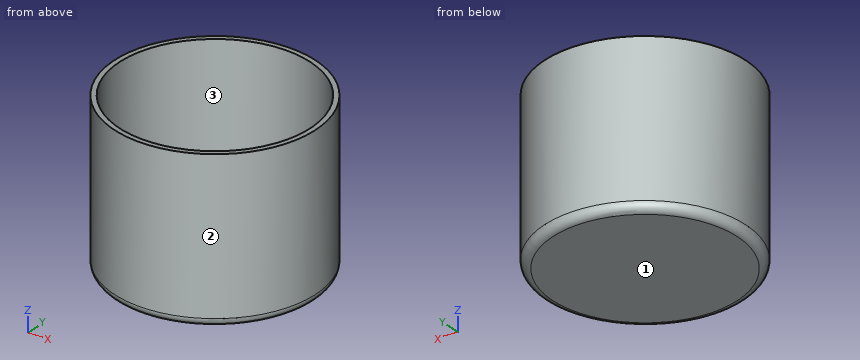
```python
from build123d import *

# Parameters (mm, degrees)
F3_DEPTH = 10


with BuildPart() as f1:
    # F0 (on Right) → F1 (revolve)
    with BuildSketch(Plane.YZ):
        with BuildLine():
            Line((0, 1.6), (0, 0))
            Line((0, 0), (29, 0))
            ThreePointArc((29, 0), (30.838478, 0.761522), (31.6, 2.6))
            Line((31.6, 2.6), (31.6, 50))
            Line((31.6, 50), (30, 50))
            Line((30, 50), (30, 2.6))
            ThreePointArc((30, 2.6), (29.707107, 1.892893), (29, 1.6))
            Line((29, 1.6), (4.2, 1.6))
            Line((4.2, 1.6), (4.2, 11.6))
            Line((4.2, 11.6), (2.6, 11.6))
            Line((2.6, 11.6), (2.6, 1.6))
            Line((2.6, 1.6), (0, 1.6))
        make_face()
    revolve(axis=Axis((0, 0, 0.8), (0, 0, 1)))

    # F2 (on face) → F3 (join, through all)
    with BuildSketch(Plane.XY.offset(11.6)):
        with BuildLine():
            ThreePointArc((1.385641, 2.2), (0, 2.6), (-1.385641, 2.2))
            Line((-1.385641, 2.2), (1.385641, 2.2))
        make_face()
    extrude(amount=-F3_DEPTH)


solid = f1.part
```
CAD build for the part. Positions are in the model's coordinates, mm. Face numbers are marked on the shaded views. Round coordinates to 2 decimals unless told otherwise and drop trailing zeros. Order: outer loops, then holes, each group sorted by start corner. A loop starts at its lowest first (then second) coordinate and runs counter-clockwise, first axis right, second up. Notation, with made-up numbers: (46, 16) - (72, 16) arc R28 ccw to (72, 50) - close; hole circle Ø3 at (88, 80). An arc over 180 degrees is marked (long way). Answer as CSV lines item,"result". Start each with the question number.
1. Saw through at C-C, the plane z = 23.5. Write the cut outline in (x, y).
2. Saw through at A-A, the plane z = 5.5. Write the cut outline in (x, y), and give its area (3 significant figures).
3. Saw through at B-B, the plane x = 0. Write the cut outline in (y, z), and give its area (3 significant figures).
4. Pin check, flat tips, straight feed: pin 1 (6 mm diameter, centred on y = -18.5, z = 40, fed in from -X); pin 2 (6.5 mm diameter, centred on x = 0, y = 0.5, fed in from +Z); pin 3 (2 mm diameter, centred on y = 4.5, z = 21.5, fed in from -X). Stop position of each tip, or through.
5. Saw through at D-D, the plane y = 0. Write the cut outline in (x, z), and give its area (3 significant figures).
6. Drill centre lines: L1, parallel to X at y = 0, z = 6; L2, parallel to Y at x = 0, z = 5; L3, parallel to X at y = 3, z = 10. Where is each one in solid material? Low to high. Write a range as [from, to].
7. Pull direction X, two halves, no side cores. Call the marked faces 1, 2 and 3: +X half, -X half, draft (parallel to the pull), parting line (faces both ways), or undercut.
Model answer:
1,outline,"circle Ø63.2 at (0, 0); hole circle Ø60 at (0, 0)"
2,outline,"circle Ø63.2 at (0, 0); circle Ø8.4 at (0, 0); hole circle Ø60 at (0, 0); hole (-1.39, 2.2) arc R2.6 ccw (long way) to (1.39, 2.2) - close"
2,area,"345 mm²"
3,outline,"(-31.6, 2.6) arc R2.6 ccw to (-29, 0) - (29, 0) arc R2.6 ccw to (31.6, 2.6) - (31.6, 50) - (30, 50) - (30, 2.6) arc R1 cw to (29, 1.6) - (4.2, 1.6) - (4.2, 11.6) - (2.2, 11.6) - (2.2, 1.6) - (-2.6, 1.6) - (-2.6, 11.6) - (-4.2, 11.6) - (-4.2, 1.6) - (-29, 1.6) arc R1 cw to (-30, 2.6) - (-30, 50) - (-31.6, 50) - close"
3,area,"290 mm²"
4,pin 1,"stops at x = -27.54"
4,pin 2,"stops at z = 11.6"
4,pin 3,"stops at x = -31.41"
5,outline,"(-31.6, 2.6) arc R2.6 ccw to (-29, 0) - (29, 0) arc R2.6 ccw to (31.6, 2.6) - (31.6, 50) - (30, 50) - (30, 2.6) arc R1 cw to (29, 1.6) - (4.2, 1.6) - (4.2, 11.6) - (2.6, 11.6) - (2.6, 1.6) - (-2.6, 1.6) - (-2.6, 11.6) - (-4.2, 11.6) - (-4.2, 1.6) - (-29, 1.6) arc R1 cw to (-30, 2.6) - (-30, 50) - (-31.6, 50) - close"
5,area,"286 mm²"
6,L1,"x = [-31.6, -30], [-4.2, -2.6], [2.6, 4.2], [30, 31.6]"
6,L2,"y = [-31.6, -30], [-4.2, -2.6], [2.2, 4.2], [30, 31.6]"
6,L3,"x = [-31.46, -29.85], [-2.94, 2.94], [29.85, 31.46]"
7,face 1,"draft"
7,face 2,"parting line"
7,face 3,"undercut"
